```python
from build123d import *

# Parameters (mm, degrees)
F0_W     = 26.4005409554
F0_H     = 18.7582788058
F0_W_2   = 54.4221671298
F0_H_2   = 12.9686864093
F0_W_3   = 31.9585492834
F0_W_4   = 55.8116771281
F0_H_3   = 18.0635303259
F1_DEPTH = 25.4


with BuildPart() as f1:
    # F0 (on Front) → F1 (new body, symmetric)
    with BuildSketch(Plane.XZ):
        Polygon((-16.0769931972, -49.6410056949), (58.9561276138, -49.6410056949), (58.9561276138, -3.3242679201), (10.3235477582, -3.3242679201), (10.3235477582, -22.0825467259), (-16.0769931972, -22.0825467259), align=None)
        Polygon((-44.0986193717, -22.0825467259), (-16.0769931972, -22.0825467259), (-16.0769931972, -3.3242679201), (10.3235477582, -3.3242679201), (10.3235477582, 11.728673242), (-44.0986193717, 11.728673242), align=None)
        with Locations((-2.8767227195, -12.703407323)):
            Rectangle(F0_W, F0_H)
        with Locations((-16.8875358067, 18.2130164467)):
            Rectangle(F0_W_2, F0_H_2)
        with Locations((26.3028223999, 18.2130164467)):
            Rectangle(F0_W_3, F0_H_2)
        with Locations((-72.0044579357, 18.2130164467)):
            Rectangle(F0_W_4, F0_H_2)
        with Locations((-16.8875358067, 33.7291248143)):
            Rectangle(F0_W_2, F0_H_3)
    extrude(amount=F1_DEPTH, both=True)


solid = f1.part
```
Could you check a few things on this model? Use its own coordinates, in mm. A direction names the side the tool comes from. Round coordinates to 2 decimals unless told otherwise and drop trailing zeros. Loops run counter-clockwise (first coordinate to the right, second up) from the corner with the lowest first, then second, coordinate; pieces in that order, holes last. Notation, with made-up numbers: (9, 20) - (44, 20) arc R34 ccw to (44, 59) - close; hole circle Ø7 at (-27.5, 47.25). An arc over 180 degrees is marked (long way). Answer as CSV lines item,"result".
1. Please list where these lines run through material, in increasing order: line 1 along Z through (x, y) = (39.5, 18); line 2 along X through (y, z) = (-1, -31); line 3 along Z through (x, y) = (-57, 4.5). Write a range as [from, to].
Filled in:
line 1,"z = [-49.64, -3.32], [11.73, 24.7]"
line 2,"x = [-16.08, 58.96]"
line 3,"z = [11.73, 24.7]"
2. For pin 1 Ø10 at (y, z) = (-3.5, -10.5) entering from -X; pin 2 Ø24.5 at (x, y) = (31, -10) entering from +Z; pin 3 Ø6.5 at (y, z) = (-7, 20) entering from +X, each with a flat end and sliding along its axis, tell me the tip position at first contact or that it passes through.
Filled in:
pin 1,"stops at x = -44.1"
pin 2,"stops at z = 24.7"
pin 3,"stops at x = 42.28"
3. We'd pull the mould along Z, two halves only. Please class faces 4 (the face through (-72, 0, 24.697)), 5 (the face through (10.324, 0, 4)), 6 (the face through (10.324, 0, 34)), 7 (the face through (35, 0, -3.324)): +Z half, -Z half, draft (parallel to the pull), parting line (faces both ways), or undercut.
Filled in:
face 4,"+Z half"
face 5,"undercut"
face 6,"draft"
face 7,"undercut"
4. I want a section at D-D on x = 47.5. List the corners of the cut face in (y, z) for me.
Filled in:
outline,"(-25.4, -49.64) - (25.4, -49.64) - (25.4, -3.32) - (-25.4, -3.32) - close"
5. I want a section at B-B on y = -20.5. List the corners of the cut face in (x, z) for me, then the cut area to 3 significant figures.
Filled in:
outline,"(-99.91, 11.73) - (-44.1, 11.73) - (-44.1, -22.08) - (-16.08, -22.08) - (-16.08, -49.64) - (58.96, -49.64) - (58.96, -3.32) - (10.32, -3.32) - (10.32, 11.73) - (42.28, 11.73) - (42.28, 24.7) - (10.32, 24.7) - (10.32, 42.76) - (-44.1, 42.76) - (-44.1, 24.7) - (-99.91, 24.7) - close"
area,"7,650 mm^2"
6. On a 3-axis mill with a long thin cutter (end or side, diameter ignored), from which of +Z, -Z, +X, -X, +Y, -Y can I reach the whole of each face in a straight line? I mean faces 1 (the face through (-44.099, 0, 34)), 2 (the face through (-72, 0, 11.729)), 3 (the face through (26, 0, 11.729)). Say none if no direction works.
Filled in:
face 1,"+Z, -X, +Y, -Y"
face 2,"-Z, -X, +Y, -Y"
face 3,"+X, +Y, -Y"
7. I want a section at A-A on x = 16. List the corners of the cut face in (y, z) for me.
Filled in:
outline,"(-25.4, -49.64) - (25.4, -49.64) - (25.4, -3.32) - (-25.4, -3.32) - close; (-25.4, 11.73) - (25.4, 11.73) - (25.4, 24.7) - (-25.4, 24.7) - close"
8. I want a section at C-C on z = 19.5. List the corners of the cut face in (x, y) for me.
Filled in:
outline,"(-99.91, -25.4) - (42.28, -25.4) - (42.28, 25.4) - (-99.91, 25.4) - close"
